from build123d import *

# Parameters (mm, degrees)
CROQUIS1_W               = 64.6
CROQUIS1_H               = 42
CROQUIS1_R               = 1.65
CROQUIS1_R_2             = 12.5
SALIENTE_EXTRUIR1_DEPTH  = 5
CROQUIS2_W               = 5
CROQUIS2_H               = 8
SALIENTE_EXTRUIR2_DEPTH  = 5
REDONDEO1_R              = 0.5
REDONDEO1_OF_SIMETR_A1_R = 0.5


with BuildPart() as part:
    # Croquis1 → Saliente-Extruir1 (new body)
    with BuildSketch(Plane.XY):
        Rectangle(CROQUIS1_W, CROQUIS1_H)
        with Locations((-15.5, 15.5)):
            Circle(CROQUIS1_R, mode=Mode.SUBTRACT)
        with Locations((15.5, 15.5)):
            Circle(CROQUIS1_R, mode=Mode.SUBTRACT)
        Circle(CROQUIS1_R_2, mode=Mode.SUBTRACT)
        with Locations((-15.5, -15.5)):
            Circle(CROQUIS1_R, mode=Mode.SUBTRACT)
        with Locations((15.5, -15.5)):
            Circle(CROQUIS1_R, mode=Mode.SUBTRACT)
    extrude(amount=SALIENTE_EXTRUIR1_DEPTH)

    # Croquis2 → Saliente-Extruir2 (add)
    with BuildSketch(Plane.ZY.offset(32.3)):
        with Locations((2.5, 12)):
            Rectangle(CROQUIS2_W, CROQUIS2_H)
        with Locations((2.5, -12)):
            Rectangle(CROQUIS2_W, CROQUIS2_H)
    saliente_extruir2 = extrude(amount=SALIENTE_EXTRUIR2_DEPTH)

    # Redondeo1
    redondeo1_edges = [part.edges().sort_by_distance(p)[0] for p in [
        (-34.8, 16, 0),
        (-34.8, 8, 0),
        (-34.8, 8, 5),
        (-34.8, 16, 5),
        (-37.3, 12, 0),
        (-37.3, 8, 2.5),
        (-37.3, 12, 5),
        (-37.3, 16, 2.5),
        (-34.8, -8, 0),
        (-34.8, -16, 0),
        (-34.8, -16, 5),
        (-34.8, -8, 5),
        (-37.3, -12, 0),
        (-37.3, -16, 2.5),
        (-37.3, -12, 5),
        (-37.3, -8, 2.5),
    ]]
    fillet(redondeo1_edges, radius=REDONDEO1_R)

    # Simetría1: Saliente-Extruir2 across plane
    add(saliente_extruir2.mirror(Plane(origin=(0, 0, 0), x_dir=(0, 0, 1), z_dir=(1, 0, 0))))

    # Redondeo1 of Simetría1
    redondeo1_of_simetr_a1_edges = [part.edges().sort_by_distance(p)[0] for p in [
        (34.8, 16, 0),
        (34.8, 8, 0),
        (34.8, 8, 5),
        (34.8, 16, 5),
        (37.3, 12, 0),
        (37.3, 8, 2.5),
        (37.3, 12, 5),
        (37.3, 16, 2.5),
        (34.8, -8, 0),
        (34.8, -16, 0),
        (34.8, -16, 5),
        (34.8, -8, 5),
        (37.3, -12, 0),
        (37.3, -16, 2.5),
        (37.3, -12, 5),
        (37.3, -8, 2.5),
    ]]
    fillet(redondeo1_of_simetr_a1_edges, radius=REDONDEO1_OF_SIMETR_A1_R)


solid = part.part
The listing builds one solid part. Answer for the finished solid, in the listing's coordinates (mm). A direction names the side the tool comes from. Coordinates: 2 decimals unless noted, no trailing zeros. Write each loop counter-clockwise with the first axis right and the second up, starting at its lowest first coordinate (ties: lowest second). Pieces come first, ordered by that corner, then holes. Notation, with made-up numbers: M 55,76.25 L 62,76.25 A14 ccw 62,86.25 Z; hole C 68.25,57.5 d5. An arc over 180 degrees is marked long. Put each result on its own line as item: value. Start each with the question number.
1. Consider line 1 (Y direction, x = 15.5, z = 2.25); line 2 (Y direction, x = 0, z = 1.15); line 3 (Y direction, x = -34, z = 4.45). Determine where each line is inside the solid, lowest interval first. Write a range as from..to.
2. A cutting plane is placed at C-C on x = 0. Write down the section's boundary in (y, z), then the cut area to 3 significant figures.
3. A cutting plane is placed at B-B on y = 0. Write down the section's boundary in (x, z), then the cut area to 3 significant figures.
4. A cutting plane is placed at A-A on x = -15.5. Write down the section's boundary in (y, z).
5. For a pull along Y with two mould halves and no side action, classify faces 5 (the flat face through (-37.3, 12, 2)), 6 (the cylindrical face through (17.024, 14.868, 2.465)), 7 (the flat face through (0, -21, 2)), 8 (the flat face through (0, 21, 2)) as pulls with the +Y half, pulls with the -Y half, needs draft (parallel to the pull), parting line crosses it, or undercut.
6. A cutting plane is placed at D-D on z = 2. Count the separate pieces of the cut face and the enclosed holes in it, then the cut area to 3 significant figures.
7. Flat-ended cylindrical pins translate along their axes: P1, Ø2.5, axis at y = -18, z = 3, coming from the +X side; P2, Ø3, axis at x = 35, z = 2, coming from the -Y side; P3, Ø2, axis at x = 34, z = 3, coming from the +Y side; P4, Ø3, axis at x = 15.5, y = 15.5, coming from the +Z side. Find the tip coordinate at first contact, or state that the pin passes through.
8. Which of the six approach directions +Z, -Z, +X, -X, +Y, -Y give full straight-line access (tool end or side, diameter ignored) to faces 1 (the flat face through (-35, -8, 2)), 2 (the flat face through (-35, -16, 2)), 3 (the flat face through (35, 16, 2)), 4 (the flat face through (35, -16, 2))?
Resolved:
1. line 1: y = -21..-17.15, -13.85..13.85, 17.15..21
1. line 2: y = -21..-12.5, 12.5..21
1. line 3: y = -16..-8, 8..16
2. outline: M -21,0 L -12.5,0 L -12.5,5 L -21,5 Z; M 12.5,0 L 21,0 L 21,5 L 12.5,5 Z
2. area: 85.0 mm2
3. outline: M -32.3,0 L -12.5,0 L -12.5,5 L -32.3,5 Z; M 12.5,0 L 32.3,0 L 32.3,5 L 12.5,5 Z
3. area: 198 mm2
4. outline: M -21,0 L -17.15,0 L -17.15,5 L -21,5 Z; M -13.85,0 L 13.85,0 L 13.85,5 L -13.85,5 Z; M 17.15,0 L 21,0 L 21,5 L 17.15,5 Z
5. face 5: needs draft
5. face 6: undercut
5. face 7: pulls with the -Y half
5. face 8: pulls with the +Y half
6. separate pieces: 1
6. enclosed holes: 5
6. area: 2,350 mm2
7. P1: stops at x = 32.3
7. P2: stops at y = -16
7. P3: stops at y = 16
7. P4: passes through
8. face 1: +Z, -Z, -X
8. face 2: +Z, -Z, -X, -Y
8. face 3: +Z, -Z, +X, +Y
8. face 4: +Z, -Z, +X, -Y
